```python
from build123d import *

# Parameters (mm, degrees)
SKETCH_W        = 54.7
SKETCH_H        = 77
PAD_DEPTH       = 53
SKETCH001_W     = 49.98
SKETCH001_H     = 71.98
POCKET_DEPTH    = 52.3
SKETCH002_R     = 5
POCKET001_DEPTH = 5
PAD001_DEPTH    = 18
SKETCH003_R     = 8
POCKET002_DEPTH = 16


with BuildPart() as part:
    # Sketch → Pad (new body)
    with BuildSketch(Plane.XY):
        with Locations((27.35, 38.5)):
            Rectangle(SKETCH_W, SKETCH_H)
    extrude(amount=PAD_DEPTH)

    # Sketch001 → Pocket (cut)
    with BuildSketch(Plane.XY):
        with Locations((27.5, 38.5)):
            Rectangle(SKETCH001_W, SKETCH001_H)
    extrude(amount=POCKET_DEPTH, mode=Mode.SUBTRACT)

    # Sketch002 → Pocket001 (cut)
    with BuildSketch(Plane.YZ):
        with Locations((20, 40)):
            Circle(SKETCH002_R)
    extrude(amount=POCKET001_DEPTH, mode=Mode.SUBTRACT)

    # Sketch004 (on DatumPlane) → Pad001 (join)
    with BuildSketch(Plane.YZ.offset(55)):
        with BuildLine():
            ThreePointArc((0, 17.8), (9.5, 27.3), (0, 36.8))
            Line((0, 36.8), (0, 17.8))
        make_face()
    extrude(amount=-PAD001_DEPTH)

    # Sketch003 (on DatumPlane) → Pocket002 (cut, symmetric)
    with BuildSketch(Plane.YZ.offset(55)):
        with Locations((0, 27.3)):
            Circle(SKETCH003_R)
    extrude(amount=POCKET002_DEPTH, both=True, mode=Mode.SUBTRACT)


solid = part.part
```
For this review, take the finished solid that the model builds, in its own axes (mm). A direction names the side the tool comes from. Round coordinates to 2 decimals unless told otherwise and drop trailing zeros. Write each loop counter-clockwise with the first axis right and the second up, starting at its lowest first coordinate (ties: lowest second). Pieces come first, ordered by that corner, then holes. Notation, with made-up numbers: M 86.5,77.25 L 133.5,77.25 A19 ccw 133.5,93.25 Z; hole C 42,6 d1. An arc over 180 degrees is marked long. One line per item, written item: value. Start each with the question number.
(1) We need section B-B (z = 48). Give the boundary of the cut face in (x, y).
(2) Machinability: for faces 4 (the cylindrical face through (44.85, 9.5, 27.13)), 5 (the flat face through (37, 5, 27)), 6 (the cylindrical face through (1.237, 19.349, 44.957)), which of the approach directions +Z, -Z, +X, -X, +Y, -Y give a long, thin tool a straight path to every point of the face, cutting with its end or side? Answer none if there is none.
(3) The part is to be moulded in two halves that separate along Y. For faces 1 (the flat face through (27, 74.49, 26)), 2 (the flat face through (28, 0, 27)), 3 (the flat face through (27, 39, 53)), say which applies: released by +Y, released by -Y, zero draft, split by the parting line, or undercut.
(4) We need section C-C (x = 18). Give the boundary of the cut face in (y, z).
(5) We need section A-A (y = 20). Give the boundary of the cut face in (x, z), and give its area (3 significant figures).
(6) We need section D-D (z = 40). Give the boundary of the cut face in (x, y).
(7) Insertion check: pin 1 (2 mm diameter, centred on y = 7, z = 26.5, fed in from -X); pin 2 (5 mm diameter, centred on y = 61.5, z = 20, fed in from +X); pin 3 (15 mm diameter, centred on x = 37, y = 29, fed in from -Z). Each pin has a flat end and moves straight along its axis. Give the tip position at first contact, or say it passes through.
(8) Wall thickness on line 1 (Y direction, x = 18, z = 23); line 2 (X direction, y = 43, z = 35.5); line 3 (Y direction, x = 1, z = 40): over which ranges is each line inside the solid? List them lowest first.
Result:
1. outline: M 0,0 L 54.7,0 L 54.7,77 L 0,77 Z; hole M 2.51,2.51 L 52.49,2.51 L 52.49,74.49 L 2.51,74.49 Z
2. face 4: none
2. face 5: -Z
2. face 6: -X
3. face 1: undercut
3. face 2: released by -Y
3. face 3: zero draft
4. outline: M 0,0 L 2.51,0 L 2.51,52.3 L 74.49,52.3 L 74.49,0 L 77,0 L 77,53 L 0,53 Z
5. outline: M 0,0 L 2.51,0 L 2.51,35 L 0,35 Z; M 0,45 L 2.51,45 L 2.51,52.3 L 52.49,52.3 L 52.49,0 L 54.7,0 L 54.7,53 L 0,53 Z
5. area: 260 mm²
6. outline: M 0,0 L 54.7,0 L 54.7,77 L 0,77 L 0,25 L 2.51,25 L 2.51,74.49 L 52.49,74.49 L 52.49,2.51 L 2.51,2.51 L 2.51,15 L 0,15 Z
7. pin 1: x = 0
7. pin 2: x = 54.7
7. pin 3: z = 52.3
8. line 1: 0 to 2.51, 74.49 to 77
8. line 2: 0 to 2.51, 52.49 to 54.7
8. line 3: 0 to 15, 25 to 77
